from build123d import *

# Parameters (mm, degrees)
SKETCH1_R           = 2.1
SKETCH1_R_2         = 1.6
SKETCH1_R_3         = 6.6
BOSS_EXTRUDE1_DEPTH = 3
CUT_EXTRUDE1_START  = -1
SKETCH2_R           = 2.6
SKETCH2_R_2         = 1.6
CUT_EXTRUDE1_DEPTH  = 1
FILLET1_R           = 0.5


with BuildPart() as part:
    # Sketch1 → Boss-Extrude1 (new body)
    with BuildSketch(Plane(origin=(0, 0, 0), x_dir=(1, 0, 0), z_dir=(0, 1, 0))):
        with BuildLine():
            ThreePointArc((-25, -5), (-30, 0), (-25, 5))
            Line((-25, 5), (-15, 5))
            ThreePointArc((-15, 5), (-7.928932188, 7.928932188), (-5, 15))
            Line((-5, 15), (-5, 25))
            ThreePointArc((-5, 25), (0, 30), (5, 25))
            Line((5, 25), (5, 15))
            ThreePointArc((5, 15), (7.928932188, 7.928932188), (15, 5))
            Line((15, 5), (25, 5))
            ThreePointArc((25, 5), (30, 0), (25, -5))
            Line((25, -5), (15, -5))
            ThreePointArc((15, -5), (7.928932188, -7.928932188), (5, -15))
            Line((5, -15), (5, -25))
            ThreePointArc((5, -25), (0, -30), (-5, -25))
            Line((-5, -25), (-5, -15))
            ThreePointArc((-5, -15), (-7.928932188, -7.928932188), (-15, -5))
            Line((-15, -5), (-25, -5))
        make_face()
        with Locations(Location((-25, 0, 0), (0, 0, 270))):
            Circle(SKETCH1_R, mode=Mode.SUBTRACT)
        with Locations(Location((0, -25, 0), (0, 0, 270))):
            Circle(SKETCH1_R, mode=Mode.SUBTRACT)
        with Locations(Location((25, 0, 0), (0, 0, 270))):
            Circle(SKETCH1_R, mode=Mode.SUBTRACT)
        with Locations(Location((0, 25, 0), (0, 0, 270))):
            Circle(SKETCH1_R, mode=Mode.SUBTRACT)
        with Locations(Location((-12.5, 0, 0), (0, 0, 270))):
            Circle(SKETCH1_R_2, mode=Mode.SUBTRACT)
        with Locations(Location((0, -12.5, 0), (0, 0, 270))):
            Circle(SKETCH1_R_2, mode=Mode.SUBTRACT)
        with Locations(Location((12.5, 0, 0), (0, 0, 270))):
            Circle(SKETCH1_R_2, mode=Mode.SUBTRACT)
        with Locations(Location((0, 12.5, 0), (0, 0, 270))):
            Circle(SKETCH1_R_2, mode=Mode.SUBTRACT)
        with Locations(Location((0, 0, 0), (0, 0, 270))):
            Circle(SKETCH1_R_3, mode=Mode.SUBTRACT)
    extrude(amount=BOSS_EXTRUDE1_DEPTH)

    # Sketch2 → Cut-Extrude1 (cut)
    # profile 1 of 4: a face of its own
    with BuildSketch(Plane(origin=(0, 3, 0), x_dir=(1, 0, 0), z_dir=(0, 1, 0)).offset(CUT_EXTRUDE1_START)):
        with Locations(Location((0, 12.5, 0), (0, 0, 270))):
            Circle(SKETCH2_R)
        with Locations(Location((0, 12.5, 0), (0, 0, 270))):
            Circle(SKETCH2_R_2, mode=Mode.SUBTRACT)
    # profile 2 of 4: a face of its own
    with BuildSketch(Plane(origin=(0, 3, 0), x_dir=(1, 0, 0), z_dir=(0, 1, 0)).offset(CUT_EXTRUDE1_START)):
        with Locations(Location((12.5, 0, 0), (0, 0, 270))):
            Circle(SKETCH2_R)
        with Locations(Location((12.5, 0, 0), (0, 0, 270))):
            Circle(SKETCH2_R_2, mode=Mode.SUBTRACT)
    # profile 3 of 4: a face of its own
    with BuildSketch(Plane(origin=(0, 3, 0), x_dir=(1, 0, 0), z_dir=(0, 1, 0)).offset(CUT_EXTRUDE1_START)):
        with Locations(Location((0, -12.5, 0), (0, 0, 270))):
            Circle(SKETCH2_R)
        with Locations(Location((0, -12.5, 0), (0, 0, 270))):
            Circle(SKETCH2_R_2, mode=Mode.SUBTRACT)
    # profile 4 of 4: a face of its own
    with BuildSketch(Plane(origin=(0, 3, 0), x_dir=(1, 0, 0), z_dir=(0, 1, 0)).offset(CUT_EXTRUDE1_START)):
        with Locations(Location((-12.5, 0, 0), (0, 0, 270))):
            Circle(SKETCH2_R)
        with Locations(Location((-12.5, 0, 0), (0, 0, 270))):
            Circle(SKETCH2_R_2, mode=Mode.SUBTRACT)
    extrude(amount=CUT_EXTRUDE1_DEPTH, mode=Mode.SUBTRACT)

    # Fillet1
    fillet1_edges = [part.edges().sort_by_distance(p)[0] for p in [
        (0, 2, -15.1),
        (12.5, 2, -2.6),
        (0, 2, 9.9),
        (-12.5, 2, -2.6),
    ]]
    fillet(fillet1_edges, radius=FILLET1_R)


solid = part.part
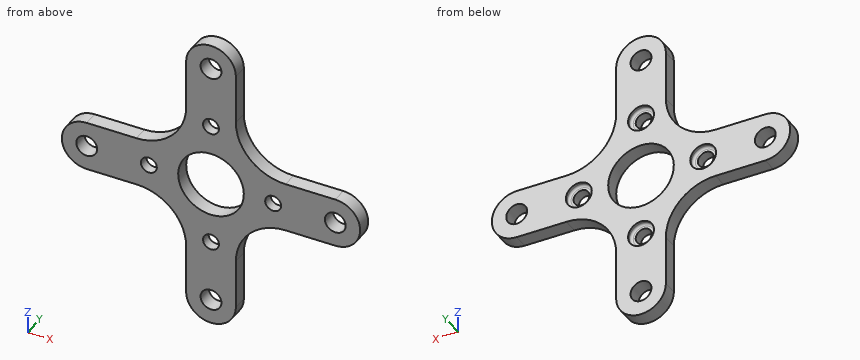
Geometry check sheet. Reference: the model listing, model coordinates, mm. Give positions to 0.01 mm unless a question says otherwise; leave off trailing zeros. Write each loop counter-clockwise with the first axis right and the second up, starting at its lowest first coordinate (ties: lowest second). Pieces come first, ordered by that corner, then holes. Notation, with made-up numbers: M 43.25,-25 L 59.25,-25 A19 ccw 59.25,2 Z; hole C 23,-1 d9. An arc over 180 degrees is marked long. One line per question, with ' | ' between items.
1. Gauge pin test, flat ends, axial feed: pin 1 (2 mm diameter, centred on x = -13, z = -1, fed in from +Y); pin 2 (1.5 mm diameter, centred on y = 1, z = 15, fed in from -X); pin 3 (0.9 mm diameter, centred on y = 1, z = -22.5, fed in from +X). Record the tip position at first contact, or that the pin passes through.
Ans:
pin 1: y = 2 | pin 2: x = -5.03 | pin 3: x = 5
2. Cross-section at C-C (y = 1.55). Count the separate pieces of the cut face and the enclosed holes in it, plus the area to 3 significant figures.
Ans:
separate pieces: 1 | enclosed holes: 9 | area: 918 mm2
3. Cross-section at A-A (z = 12.5). Enter the section's corners in (x, y), plus the area to 3 significant figures.
Ans:
outline: M -5.32,0 L -1.6,0 L -1.6,2 L -2.1,2 A0.5 cw -2.6,2.5 L -2.6,3 L -5.32,3 Z; M 1.6,0 L 5.32,0 L 5.32,3 L 2.6,3 L 2.6,2.5 A0.5 cw 2.1,2 L 1.6,2 Z | area: 20.4 mm2
4. Scan lines: line 1 along X through (y, z) = (1.6, 4); line 2 along Z through (x, y) = (-24, 1.45); line 3 along X through (y, z) = (2.8, 12.5). Record each from-to range of solid material in increasing order. Write a range as from..to.
Ans:
line 1: -28..-5.25, 5.25..28 | line 2: -5..-1.85, 1.85..5 | line 3: -5.32..-2.6, 2.6..5.32
5. Cross-section at B-B (x = -12.5). Enter the section's corners in (y, z).
Ans:
outline: M 0,-5.32 L 3,-5.32 L 3,-2.6 L 2.5,-2.6 A0.5 cw 2,-2.1 L 2,-1.6 L 0,-1.6 Z; M 0,1.6 L 2,1.6 L 2,2.1 A0.5 cw 2.5,2.6 L 3,2.6 L 3,5.32 L 0,5.32 Z
